The listing builds one solid part. Answer for the finished solid, in the listing's coordinates (mm). A direction names the side the tool comes from. Coordinates: 2 decimals unless noted, no trailing zeros. Loops run counter-clockwise (first coordinate to the right, second up) from the corner with the lowest first, then second, coordinate; pieces in that order, holes last. Notation, with made-up numbers: (6.5, 67) - (51.5, 67) arc R19 cw to (51.5, 87) - close; hole circle Ø9 at (6.5, -29). An arc over 180 degrees is marked (long way). One line per question, with ' | ' between items.
from build123d import *

# Parameters (mm, degrees)
Y_KSEKLIK_EKSTR_ZYON1_DEPTH = 20
RADYUS1_R                   = 1
KES_EKSTR_ZYON1_REACH       = 59.775
IZIM2_R                     = 2
IZIM3_R                     = 2
Y_KSEKLIK_EKSTR_ZYON2_DEPTH = 6


with BuildPart() as part:
    # Çizim1 → Yükseklik-Ekstrüzyon1 (new body)
    with BuildSketch(Plane.XY):
        Polygon((0, 0), (40, 0), (40, 25), (47, 25), (47, 27), (40, 27), (40, 40), (0, 40), (0, 27), (-7, 27), (-7, 25), (0, 25), align=None)
    extrude(amount=Y_KSEKLIK_EKSTR_ZYON1_DEPTH)

    # Radyus1
    radyus1_edges = [part.edges().sort_by_distance(p)[0] for p in [
        (-7, 26, 0),
        (47, 26, 0),
        (47, 26, 20),
        (-7, 26, 20),
    ]]
    fillet(radyus1_edges, radius=RADYUS1_R)

    # Çizim2 → Kes-Ekstrüzyon1 (cut, up to next)
    with BuildSketch(Plane(origin=(0, 27, 0), x_dir=(1, 0, 0), z_dir=(0, 1, 0)), mode=Mode.PRIVATE) as kes_ekstr_zyon1_sk1:
        with Locations(Location((-3.5, -5, 0), (0, 0, 270))):
            Circle(IZIM2_R)
    kes_ekstr_zyon1_tool1 = extrude(kes_ekstr_zyon1_sk1.sketch, amount=-KES_EKSTR_ZYON1_REACH, mode=Mode.PRIVATE) & part.part
    # Çizim2 → Kes-Ekstrüzyon1 (cut, up to next)
    with BuildSketch(Plane(origin=(0, 27, 0), x_dir=(1, 0, 0), z_dir=(0, 1, 0)), mode=Mode.PRIVATE) as kes_ekstr_zyon1_sk2:
        with Locations(Location((-3.5, -15, 0), (0, 0, 270))):
            Circle(IZIM2_R)
    kes_ekstr_zyon1_tool2 = extrude(kes_ekstr_zyon1_sk2.sketch, amount=-KES_EKSTR_ZYON1_REACH, mode=Mode.PRIVATE) & part.part
    # Çizim2 → Kes-Ekstrüzyon1 (cut, up to next)
    with BuildSketch(Plane(origin=(0, 27, 0), x_dir=(1, 0, 0), z_dir=(0, 1, 0)), mode=Mode.PRIVATE) as kes_ekstr_zyon1_sk3:
        with Locations(Location((43.5, -5, 0), (0, 0, 270))):
            Circle(IZIM2_R)
    kes_ekstr_zyon1_tool3 = extrude(kes_ekstr_zyon1_sk3.sketch, amount=-KES_EKSTR_ZYON1_REACH, mode=Mode.PRIVATE) & part.part
    # Çizim2 → Kes-Ekstrüzyon1 (cut, up to next)
    with BuildSketch(Plane(origin=(0, 27, 0), x_dir=(1, 0, 0), z_dir=(0, 1, 0)), mode=Mode.PRIVATE) as kes_ekstr_zyon1_sk4:
        with Locations(Location((43.5, -15, 0), (0, 0, 270))):
            Circle(IZIM2_R)
    kes_ekstr_zyon1_tool4 = extrude(kes_ekstr_zyon1_sk4.sketch, amount=-KES_EKSTR_ZYON1_REACH, mode=Mode.PRIVATE) & part.part
    add(kes_ekstr_zyon1_tool1.solids().sort_by_distance((-3.5, 27, 5))[0], mode=Mode.SUBTRACT)
    add(kes_ekstr_zyon1_tool2.solids().sort_by_distance((-3.5, 27, 15))[0], mode=Mode.SUBTRACT)
    add(kes_ekstr_zyon1_tool3.solids().sort_by_distance((43.5, 27, 5))[0], mode=Mode.SUBTRACT)
    add(kes_ekstr_zyon1_tool4.solids().sort_by_distance((43.5, 27, 15))[0], mode=Mode.SUBTRACT)

    # Çizim3 → Yükseklik-Ekstrüzyon2 (add)
    with BuildSketch(Plane(origin=(0, 40, 0), x_dir=(1, 0, 0), z_dir=(0, 1, 0))):
        with Locations(Location((10, -10, 0), (0, 0, 90))):
            Circle(IZIM3_R)
    extrude(amount=Y_KSEKLIK_EKSTR_ZYON2_DEPTH)


solid = part.part
Item 1: Find section A-A, the plane x = 43.5. Write down the section's boundary in (y, z), plus the area to 3 significant figures.
Taken from the geometry:
outline: (25, 0) - (27, 0) - (27, 3) - (25, 3) - close; (25, 7) - (27, 7) - (27, 13) - (25, 13) - close; (25, 17) - (27, 17) - (27, 20) - (25, 20) - close | area: 24.0 mm2
Item 2: Find section B-B, the plane z = 5. Write down the section's boundary in (x, y), plus the area to 3 significant figures.
Taken from the geometry:
outline: (-7, 25) - (-5.5, 25) - (-5.5, 27) - (-7, 27) - close; (-1.5, 25) - (0, 25) - (0, 0) - (40, 0) - (40, 25) - (41.5, 25) - (41.5, 27) - (40, 27) - (40, 40) - (0, 40) - (0, 27) - (-1.5, 27) - close; (45.5, 25) - (47, 25) - (47, 27) - (45.5, 27) - close | area: 1,610 mm2
Item 3: Find the intervals of material crossed by line 1 (X direction, y = 26, z = 15); line 2 (Z direction, x = 43, y = 26); line 3 (Y direction, x = 26.5, z = 17.75), in increasing order. Write a range as [from, to].
Taken from the geometry:
line 1: x = [-7, -5.5], [-1.5, 41.5], [45.5, 47] | line 2: z = [0, 3.06], [6.94, 13.06], [16.94, 20] | line 3: y = [0, 40]
Item 4: Find section D-D, the plane x = 10. Write down the section's boundary in (y, z), plus the area to 3 significant figures.
Taken from the geometry:
outline: (0, 0) - (40, 0) - (40, 8) - (46, 8) - (46, 12) - (40, 12) - (40, 20) - (0, 20) - close | area: 824 mm2
Item 5: The mould has two halves that part along X. Classify faces 1 (the face through (41.548, 26.014, 4.566)), 2 (the face through (20, 20, 0)), 3 (the face through (8, 43, 10)): pulls with the +X half, pulls with the -X half, needs draft (parallel to the pull), parting line crosses it, or undercut.
Taken from the geometry:
face 1: undercut | face 2: needs draft | face 3: parting line crosses it
Item 6: Which of the six approach directions +Z, -Z, +X, -X, +Y, -Y give full straight-line access (tool end or side, diameter ignored) to faces 4 (the face through (43, 25, 10)), 5 (the face through (44, 27, 10)), 6 (the face through (-3, 27, 10)), 7 (the face through (0, 13, 10))?
Taken from the geometry:
face 4: +Z, -Z, +X, -Y | face 5: +Z, -Z, +X, +Y | face 6: +Z, -Z, -X, +Y | face 7: +Z, -Z, -X, -Y
Item 7: Find section C-C, the plane z = 10. Write down the section's boundary in (x, y).
Taken from the geometry:
outline: (-7, 25) - (0, 25) - (0, 0) - (40, 0) - (40, 25) - (47, 25) - (47, 27) - (40, 27) - (40, 40) - (12, 40) - (12, 46) - (8, 46) - (8, 40) - (0, 40) - (0, 27) - (-7, 27) - close
Item 8: Each of these flat-tipped pins is pushed along its axis until it touches: pin 1 Ø10 at (y, z) = (8.5, 14.5) entering from +X; pin 2 Ø10 at (x, z) = (37, 7) entering from +Y; pin 3 Ø3.5 at (x, z) = (43, 10) entering from -Y; pin 4 Ø3.5 at (x, z) = (-3.5, 5) entering from -Y. Where does it stop, or does it pass through?
Taken from the geometry:
pin 1: stops at x = 40 | pin 2: stops at y = 40 | pin 3: stops at y = 25 | pin 4: passes through
